Autodesk Inventor part; units mm, degrees
ref_plane "Work Plane1" through (29, 0, 0) normal (0, -1, 0) x (1, 0, 0)
ref_plane "YZ Plane" through (0, 0, 0) normal (1, 0, 0) x (0, 1, 0)
ref_plane "XZ Plane" through (0, 0, 0) normal (0, 1, 0) x (-1, 0, 0)
sketch "Sketch1" plane through (0, 0, 0) normal (0, 0, 1) x (1, 0, 0)
  line L0 (-0.6667, 0) -> (14, 0)
  line L1 (14, 0) -> (14, 1.5)
  line L2 (14, 1.5) -> (1, 1.5)
  line L3 (1, 1.5) -> (0.6932, 1.5)
  line L4 (0.6932, 1.5) -> (0, 1.5)
  line L5 (0, 1.5) -> (0, 2.75)
  line L6 (0, 2.75) -> (-3, 2.75)
  line L7 (-3, 2.75) -> (-3, 1.4434)
  line L8 (-3, 1.4434) -> (-1.5, 1.4434)
  line L9 (-1.5, 1.4434) -> (-0.6667, 0)
  line L10 (-6.8, 0) -> (19.8, 0)
  line L11 (0, -0.55) -> (0, 3.3)
  line L12 (1, 1.5) -> (0, 1.5) construction
  dimension "d1" = 13
  dimension "d2" = 0.3068
  dimension "d3" = 3
  dimension "d4" = 1.5
  dimension "d5" = 60
  dimension "d6" = 3
  dimension "d7" = 3
  dimension "d8" = 2.8868
  dimension "d9" = 5.5
  dimension "d26" = 14
revolve "Body" add sketch "Sketch1" angle 360 about axis through (-0.6667, 0, 0) along (1, 0, 0)
sketch "Sketch2" plane through (-3, 0, 0) normal (-1, 0, 0) x (0, 0, 1)
  circle A0 centre (0, 0) radius 1.4434
  line L0 (0, -3.85) -> (0, 3.85)
  line L1 (-3.85, 0) -> (3.85, 0)
  line L2 (1.4434, 0) -> (0.7217, -1.25)
  line L3 (0.7217, -1.25) -> (-0.7217, -1.25)
  line L4 (-0.7217, -1.25) -> (-1.4434, 0)
  line L5 (-1.4434, 0) -> (-0.7217, 1.25)
  line L6 (-0.7217, 1.25) -> (0.7217, 1.25)
  line L7 (0.7217, 1.25) -> (1.4434, 0)
extrude "Slot" add sketch "Sketch2" against normal up to next contours L7 A0 | A0 L2 | L6 L0 A0 | A0 L0 L3 | L0 L6 A0 | A0 L3 L0 | L4 A0 | A0 L5
fillet "Fillet1" radius 0.3 1 edges at (-3, -2.75, 0)
thread "Thread"
chamfer "Chamfer1" distance 0.3067 distance2 0.3067 1 edges at (14, -1.5, 0) measured on face at (14, 0.5539, 0.4443)
ref_plane "Work Plane1" through (29, 0, 0) normal (0, -1, 0) x (1, 0, 0)
fillet "Fillet2" radius 0.1 1 edges at (0, -1.5, 0)
equation "\"d1\" = GEL"
equation "\"d3\" = KOH"
equation "\"d4\" = INTI"
equation "\"d6\" = GD"
equation "\"d7\" = BDM"
equation "\"d8\" = 1.1547 * SW"
equation "\"d9\" = KOD"
equation "\"d26\" = NLG"
equation "\"d30\" = R"
equation "\"d17\" = RR"
equation "\"d13\" = GEL"
equation "\"d15\" = -0.5 * SPD + 0.5 * GD"
equation "\"d16\" = GUL"
equation "\"GD\" = NND"
equation "\"NLG\" = 14"
equation "\"GEL\" = 13"
equation "\"KOD\" = 5.5"
equation "\"KOH\" = 3"
equation "\"INTI\" = 1.5"
equation "\"GAL\" = 0.61345 * PTC"
equation "\"GUL\" = 0.61345 * PTC"
equation "\"BDM\" = NND"
equation "\"SW\" = 2.5"
equation "\"RR\" = 0.3"
equation "\"SPD\" = 2.38655"
equation "\"R\" = 0.1"
equation "\"TOA\" = 30deg"
equation "\"THREADDIA\" = 3"
equation "\"PTC\" = 0.5"
equation "\"NND\" = 3"
equation "\"E0\" = 1.155 * SW"
equation "\"GD1\" = THREADDIA - 1.2269 * PTC"
properties material "Steel, Mild"
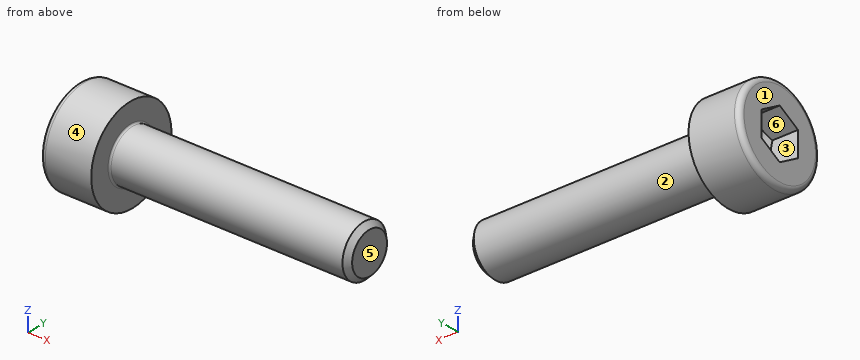
For this review, take the finished solid that the model builds, in its own axes (mm). Face numbers are marked on the shaded views. A direction names the side the tool comes from. Round coordinates to 2 decimals unless told otherwise and drop trailing zeros. Order: outer loops, then holes, each group sorted by start corner. A loop starts at its lowest first (then second) coordinate and runs counter-clockwise, first axis right, second up. Notation, with made-up numbers: M 7,40 L 45,40 A22 cw 45,64 Z; hole C 69,5 d10. An arc over 180 degrees is marked long. Use a Markdown table: item, result. Add a question column.
Item 1: Mouldability with a two-part tool opening along Y and no side actions: class the marked faces 4, 5 and 6 as released by +Y, released by -Y, zero draft, split by the parting line, or undercut.
Item 2: Tool access review of the marked faces 1, 2 and 3: name each direction out of +Z, -Z, +X, -X, +Y, -Y from which nothing blocks a thin tool from reaching the whole face with its end or side.
Item 3: To check wall thickness, follow line 1 along Z through (x, y) = (7.5, -0.4); line 2 along X through (y, z) = (1.75, -0.8); line 3 along Y through (x, z) = (8, -0.1). State the ranges of each line that lie inside material, in increasing order.
Item 4: Insertion check: pin 1 (2 mm diameter, centred on x = 7.5, y = 0, fed in from +Z); pin 2 (1.5 mm diameter, centred on x = 7, z = 1.5, fed in from -Y). Each pin has a flat end and moves straight along its axis. Give the tip position at first contact, or say it passes through.
Item 5: Add section A-A, the plane x = 4. Give the boundary of the cut face in (y, z).
Geometry results:
| question | item | result |
|---|---|---|
| 1 | face 4 | split by the parting line |
| 1 | face 5 | zero draft |
| 1 | face 6 | undercut |
| 2 | face 1 | +Z, -Z, -X, +Y, -Y |
| 2 | face 2 | +X |
| 2 | face 3 | -X |
| 3 | line 1 | z = -1.45 to 1.45 |
| 3 | line 2 | x = -3 to 0 |
| 3 | line 3 | y = -1.5 to 1.5 |
| 4 | pin 1 | stops at z = 1.5 |
| 4 | pin 2 | stops at y = -1.3 |
| 5 | outline | C 0,0 d3 |
